Can you work these out from the model? Positions are in its coordinate system, mm. Round coordinates to 2 decimals unless told otherwise and drop trailing zeros. Write each loop counter-clockwise with the first axis right and the second up, starting at its lowest first coordinate (ties: lowest second). Pieces come first, ordered by that corner, then holes. Notation, with made-up numbers: M 3,-27 L 9,-27 A12 ccw 9,-17 Z; hole C 27.25,-12.75 d6. An arc over 180 degrees is marked long. Answer in a Markdown table with one row per item. Add a question column.
(1) Suppose I cut it at C-C, the plane y = 116.5. Write out the boundary of the cut face in (x, z).
(2) Suppose I cut it at D-D, the plane y = 5. Write out the boundary of the cut face in (x, z).
(3) Suppose I cut it at A-A, the plane y = 76.5. Write out the boundary of the cut face in (x, z), then the cut area to 3 significant figures.
(4) Suppose I cut it at B-B, the plane z = 14. Count the separate pieces of the cut face and the enclosed holes in it, then the cut area to 3 significant figures.
(5) If we mould it in two halves opening along Y, with no side actions, what happens to faces 1 (the face through (-1.398, 140.313, 9.86)), 2 (the face through (-1.6, 74, 10)), 3 (the face through (-26, 45, 0))? For each: released by +Y, released by -Y, zero draft, split by the parting line, or undercut.
(6) If I drill on probe 1 along X at (y, z) = (74.5, 5.75); probe 2 along X at (y, z) = (45, 7.5); probe 3 along X at (y, z) = (121, 6), over which ranges is the centre line in solid material (lowest first)?
(7) I'm going to push flat-ended pins straight in: pin 1 (11.5 mm diameter, centred on y = 71, z = 13.5, fed in from -X); pin 2 (3 mm diameter, centred on x = -5, y = 5, fed in from +Z); pin 3 (7 mm diameter, centred on y = 13.5, z = 5.5, fed in from -X); pin 4 (8 mm diameter, centred on x = -20.5, z = 17.5, fed in from +Y). Where does each tip first touch, or does it pass through?
from build123d import *

# Parameters (mm, degrees)
BOSS_EXTRUDE4_DEPTH = 20
SKETCH12_R          = 1.65
CUT_EXTRUDE1_DEPTH  = 149.790905386
CUT_EXTRUDE2_START  = -20
CUT_EXTRUDE2_DEPTH  = 20
CUT_EXTRUDE3_START  = -30
CUT_EXTRUDE3_DEPTH  = 30
BOSS_EXTRUDE5_DEPTH = 20
CIRPATTERN1_COUNT   = 6
CIRPATTERN1_ANGLE   = 30
LPATTERN2_COUNT     = 3
LPATTERN2_PITCH     = 10
BOSS_EXTRUDE6_DEPTH = 20
LPATTERN3_COUNT     = 3
LPATTERN3_PITCH     = 15
CUT_EXTRUDE4_START  = -20
CUT_EXTRUDE4_DEPTH  = 20


with BuildPart() as part:
    # Sketch5 → Boss-Extrude4 (new body)
    with BuildSketch(Plane.XY):
        with BuildLine():
            Line((0, 0), (0, 138.405603612))
            ThreePointArc((0, 138.405603612), (-1.431938837, 140.323234054), (-3.677306515, 139.494934991))
            ThreePointArc((-3.677306515, 139.494934991), (-34.45212059, 72.743387818), (-45, 0))
            Line((-45, 0), (0, 0))
        make_face()
        with BuildLine():
            Line((-1.6, 10), (-40.801596678, 10))
            ThreePointArc((-40.801596678, 10), (-30.171322984, 73.09445494), (-4, 131.480881584))
            ThreePointArc((-4, 131.480881584), (-2.54422163, 132.052107892), (-1.6, 130.805498221))
            Line((-1.6, 130.805498221), (-1.6, 10))
        make_face(mode=Mode.SUBTRACT)
    extrude(amount=BOSS_EXTRUDE4_DEPTH)

    # Sketch12 → Cut-Extrude1 (cut, through all)
    with BuildSketch(Plane.XY.offset(20)):
        with Locations((-40, 5)):
            Circle(SKETCH12_R)
        with Locations((-22.5, 5)):
            Circle(SKETCH12_R)
        with Locations((-5, 5)):
            Circle(SKETCH12_R)
    extrude(amount=-CUT_EXTRUDE1_DEPTH, mode=Mode.SUBTRACT)

    # Sketch17 → Cut-Extrude2 (cut)
    with BuildSketch(Plane.XY.offset(20).offset(CUT_EXTRUDE2_START)):
        Polygon((-109.129206393, -31.174044695), (890.870793607, -18.386269912), (884.13367644, 508.454191469), (-120.638203698, 868.825955305), (-717.462714608, 272.001444394), align=None)
        with BuildLine():
            Line((-45, 0), (0, 0))
            Line((0, 0), (0, 138.405603612))
            ThreePointArc((0, 138.405603612), (-0.890765175, 140.069814567), (-2.769598102, 140.25160436))
            ThreePointArc((-2.769598102, 140.25160436), (-57.041683198, 80.109492203), (-45, 0))
        make_face(mode=Mode.SUBTRACT)
    extrude(amount=CUT_EXTRUDE2_DEPTH, mode=Mode.SUBTRACT)

    # Sketch18 → Cut-Extrude3 (cut)
    with BuildSketch(Plane.XY.offset(20).offset(CUT_EXTRUDE3_START)):
        Polygon((10.567687301, -7.152622061), (26.572035637, 318.782087337), (-234.729728554, 306.471050155), (-205.798791176, -46.855716973), align=None)
        with BuildLine():
            Line((-45, 0), (0, 0))
            Line((0, 0), (0, 138.405603612))
            ThreePointArc((0, 138.405603612), (-1.431938837, 140.323234054), (-3.677306515, 139.494934991))
            ThreePointArc((-3.677306515, 139.494934991), (-34.45212059, 72.743387818), (-45, 0))
        make_face(mode=Mode.SUBTRACT)
    extrude(amount=CUT_EXTRUDE3_DEPTH, mode=Mode.SUBTRACT)

    # Sketch14 → Boss-Extrude5 (add)
    with BuildSketch(Plane.XY.offset(20)):
        Polygon((48.4, 10), (-114.101488266, 62.799934205), (-113.483454278, 64.702047237), (49.018033989, 11.902113033), align=None)
    boss_extrude5 = extrude(amount=-BOSS_EXTRUDE5_DEPTH)

    # CirPattern1: Boss-Extrude5 ×6 about axis
    cirpattern1_axis = Axis((49.018033989, 11.902113033, 0), (0, 0, -1))
    for i in range(1, CIRPATTERN1_COUNT):
        add(boss_extrude5.rotate(cirpattern1_axis, i * CIRPATTERN1_ANGLE / (CIRPATTERN1_COUNT - 1)))

    # LPattern2: Boss-Extrude5 ×3
    with Locations(*[(0, -i * LPATTERN2_PITCH, 0) for i in range(1, LPATTERN2_COUNT)]):
        add(boss_extrude5)

    # Sketch19 → Boss-Extrude6 (add)
    with BuildSketch(Plane.XY.offset(20)):
        Polygon((-1.6, 78.758131997), (-60.025016892, 143.645686936), (-58.538727241, 144.983948149), (-0.113710349, 80.096393209), align=None)
    boss_extrude6 = extrude(amount=-BOSS_EXTRUDE6_DEPTH)

    # LPattern3: Boss-Extrude6 ×3
    with Locations(*[(0, i * LPATTERN3_PITCH, 0) for i in range(1, LPATTERN3_COUNT)]):
        add(boss_extrude6)

    # Sketch20 → Cut-Extrude4 (cut)
    with BuildSketch(Plane.XY.offset(20).offset(CUT_EXTRUDE4_START)):
        Polygon((77.475806055, -29.017161833), (-265.551297842, 6.523481062), (-137.36538358, 367.52057294), (154.147754773, 113.145409747), align=None)
        with BuildLine():
            Line((-45, 0), (0, 0))
            Line((0, 0), (0, 138.405603612))
            ThreePointArc((0, 138.405603612), (-1.431938837, 140.323234054), (-3.677306515, 139.494934991))
            ThreePointArc((-3.677306515, 139.494934991), (-34.45212059, 72.743387818), (-45, 0))
        make_face(mode=Mode.SUBTRACT)
    extrude(amount=CUT_EXTRUDE4_DEPTH, mode=Mode.SUBTRACT)


solid = part.part
Calculated:
| question | item | result |
|---|---|---|
| 1 | outline | M -16.97,0 L -12.47,0 L -12.47,20 L -16.97,20 Z; M -8.57,0 L -5.88,0 L -5.88,20 L -8.57,20 Z; M -1.6,0 L 0,0 L 0,20 L -1.6,20 Z |
| 2 | outline | M -44.95,0 L -41.65,0 L -41.65,20 L -44.95,20 Z; M -38.35,0 L -24.15,0 L -24.15,20 L -38.35,20 Z; M -20.85,0 L -6.65,0 L -6.65,20 L -20.85,20 Z; M -3.35,0 L 0,0 L 0,20 L -3.35,20 Z |
| 3 | outline | M -33.31,0 L -29.11,0 L -29.11,20 L -33.31,20 Z; M -25.71,0 L -22.73,0 L -22.73,20 L -25.71,20 Z; M -11.84,0 L -9.15,0 L -9.15,20 L -11.84,20 Z; M -1.6,0 L 0,0 L 0,20 L -1.6,20 Z |
| 3 | area | 229 mm² |
| 4 | separate pieces | 1 |
| 4 | enclosed holes | 15 |
| 4 | area | 1,890 mm² |
| 5 | face 1 | released by +Y |
| 5 | face 2 | undercut |
| 5 | face 3 | zero draft |
| 6 | probe 1 | -33.92 to -29.74, -23.49 to -20.5, -10.04 to -7.35, -1.6 to 0 |
| 6 | probe 2 | -41.02 to -36.95, -30.24 to -25.32, -12.31 to -8.31, -1.6 to 0 |
| 6 | probe 3 | -14.61 to -9.93, -1.6 to 0 |
| 7 | pin 1 | x = -36.55 |
| 7 | pin 2 | through |
| 7 | pin 3 | x = -44.8 |
| 7 | pin 4 | y = 117.41 |
